from build123d import *

# Parameters (mm, degrees)
SKETCH1_W                 = 75
SKETCH1_H                 = 40
SKETCH1_R                 = 5
SKETCH1_R_2               = 1.7
SKETCH1_W_2               = 10
SKETCH1_H_2               = 20
BOSS_EXTRUDE1_DEPTH       = 3
CUT_EXTRUDE1_DEPTH        = 43.605750786
CUT_EXTRUDE1_DEPTH_BACK   = 43.605750786
SKETCH2_W                 = 67
SKETCH2_H                 = 28
BOSS_EXTRUDE3_DEPTH       = 110
BOSS_EXTRUDE3_DEPTH_BACK  = 3
SKETCH6_W                 = 67
SKETCH6_H                 = 11
CUT_EXTRUDE4_DEPTH        = 122.372360939
SKETCH7_W                 = 70
SKETCH7_H                 = 37
BOSS_EXTRUDE4_DEPTH       = 45
SKETCH8_W                 = 45
SKETCH8_H                 = 62
CUT_EXTRUDE6_DEPTH        = 29
SKETCH11_W                = 45
SKETCH11_H                = 4
CUT_EXTRUDE9_DEPTH        = 157.445677473
SKETCH9_W                 = 38
SKETCH9_H                 = 28.5
CUT_EXTRUDE10_DEPTH       = 204.024629048
SKETCH13_W                = 5
SKETCH13_H                = 38
BOSS_EXTRUDE5_DEPTH       = 32
SKETCH14_R                = 5
SKETCH14_R_2              = 1.7
CUT_EXTRUDE11_DEPTH       = 32
SKETCH15_W                = 165
SKETCH15_H                = 70
SKETCH15_W_2              = 157
SKETCH15_H_2              = 62
BOSS_EXTRUDE6_DEPTH       = 3
SKETCH16_W                = 20
SKETCH16_H                = 4.820648258
CUT_EXTRUDE12_DEPTH       = 159.626132778
SKETCH18_R                = 5
CUT_EXTRUDE14_DEPTH       = 159.626132778
MIRROR6_COPY_1_SKETCH_W   = 5
MIRROR6_COPY_1_SKETCH_H   = 38
MIRROR6_COPY_1_DEPTH      = 32
MIRROR6_COPY_2_SKETCH_R   = 5
MIRROR6_COPY_2_SKETCH_R_2 = 1.7
MIRROR6_COPY_2_DEPTH      = 32
SKETCH19_W                = 38
SKETCH19_H                = 3.5
CUT_EXTRUDE15_DEPTH       = 10
SKETCH20_R                = 1.2
CUT_EXTRUDE16_DEPTH       = 10
SKETCH21_W                = 10
SKETCH21_H                = 80
CUT_EXTRUDE17_DEPTH       = 184.330984833
SKETCH22_W                = 55
SKETCH22_H                = 80
CUT_EXTRUDE18_DEPTH       = 184.330984833
SKETCH23_W                = 67
SKETCH23_H                = 62
BOSS_EXTRUDE7_DEPTH       = 3
SKETCH24_R                = 10
SKETCH24_R_2              = 2.75
CUT_EXTRUDE19_DEPTH       = 111.707949127
SKETCH25_W                = 38
SKETCH25_H                = 64
CUT_EXTRUDE20_DEPTH       = 115
SKETCH26_W                = 49
SKETCH26_H                = 35
CUT_EXTRUDE21_DEPTH       = 32
SKETCH27_R                = 4.4
BOSS_EXTRUDE8_DEPTH       = 46


with BuildPart() as part:
    # Sketch1 → Boss-Extrude1 (new body)
    with BuildSketch(Plane(origin=(0, 0, 0), x_dir=(1, 0, 0), z_dir=(0, 1, 0))):
        Rectangle(SKETCH1_W, SKETCH1_H)
        with Locations(Location((-21, 0, 0), (0, 0, 270))):
            Circle(SKETCH1_R, mode=Mode.SUBTRACT)
        with Locations(Location((-30, 8.25, 0), (0, 0, 270))):
            Circle(SKETCH1_R_2, mode=Mode.SUBTRACT)
        with Locations(Location((-12, 8.25, 0), (0, 0, 270))):
            Circle(SKETCH1_R_2, mode=Mode.SUBTRACT)
        with Locations(Location((-12, -8.25, 0), (0, 0, 270))):
            Circle(SKETCH1_R_2, mode=Mode.SUBTRACT)
        with Locations(Location((-30, -8.25, 0), (0, 0, 270))):
            Circle(SKETCH1_R_2, mode=Mode.SUBTRACT)
        with Locations(Location((12, 8.25, 0), (0, 0, 90))):
            Circle(SKETCH1_R_2, mode=Mode.SUBTRACT)
        with Locations(Location((12, -8.25, 0), (0, 0, 90))):
            Circle(SKETCH1_R_2, mode=Mode.SUBTRACT)
        with Locations(Location((21, 0, 0), (0, 0, 90))):
            Circle(SKETCH1_R, mode=Mode.SUBTRACT)
        with Locations(Location((30, -8.25, 0), (0, 0, 90))):
            Circle(SKETCH1_R_2, mode=Mode.SUBTRACT)
        with Locations(Location((30, 8.25, 0), (0, 0, 90))):
            Circle(SKETCH1_R_2, mode=Mode.SUBTRACT)
        Rectangle(SKETCH1_W_2, SKETCH1_H_2, mode=Mode.SUBTRACT)
    extrude(amount=BOSS_EXTRUDE1_DEPTH)

    # Sketch2 → Cut-Extrude1 (cut, two sides: drawn at the far end of the back side and taken through both)
    with BuildSketch(Plane(origin=(0, 3, 0), x_dir=(1, 0, 0), z_dir=(0, 1, 0)).offset(-CUT_EXTRUDE1_DEPTH_BACK)):
        Rectangle(SKETCH2_W, SKETCH2_H)
    extrude(amount=CUT_EXTRUDE1_DEPTH + CUT_EXTRUDE1_DEPTH_BACK, mode=Mode.SUBTRACT)

    # Sketch3 → Boss-Extrude3 (add, two sides: drawn at the far end of the back side and taken through both)
    with BuildSketch(Plane(origin=(0, 3, 0), x_dir=(1, 0, 0), z_dir=(0, 1, 0)).offset(-BOSS_EXTRUDE3_DEPTH_BACK)):
        Polygon((37.5, -35), (37.5, -20), (33.5, -20), (-33.5, -20), (-37.5, -20), (-37.5, -35), align=None)
        Polygon((33.5, 20), (37.5, 20), (37.5, 35), (-37.5, 35), (-37.5, 20), (-33.5, 20), align=None)
        Polygon((37.5, -20), (37.5, 20), (33.5, 20), (33.5, 14), (33.5, -14), (33.5, -20), align=None)
        Polygon((-33.5, 14), (-33.5, 20), (-37.5, 20), (-37.5, -20), (-33.5, -20), (-33.5, -14), align=None)
    extrude(amount=BOSS_EXTRUDE3_DEPTH + BOSS_EXTRUDE3_DEPTH_BACK)

    # Sketch6 → Cut-Extrude4 (cut, through all)
    with BuildSketch(Plane(origin=(0, 3, 0), x_dir=(1, 0, 0), z_dir=(0, 1, 0))):
        with Locations((0, -25.5)):
            Rectangle(SKETCH6_W, SKETCH6_H)
        with Locations((0, 25.5)):
            Rectangle(SKETCH6_W, SKETCH6_H)
    extrude(amount=CUT_EXTRUDE4_DEPTH, mode=Mode.SUBTRACT)

    # Sketch7 → Boss-Extrude4 (add)
    with BuildSketch(Plane.ZY.offset(37.5)):
        with Locations((0, 94.5)):
            Rectangle(SKETCH7_W, SKETCH7_H)
    boss_extrude4 = extrude(amount=BOSS_EXTRUDE4_DEPTH)

    # Mirror2: Boss-Extrude4 across plane
    add(boss_extrude4.mirror(Plane(origin=(0, 0, 0), x_dir=(0, 0, 1), z_dir=(1, 0, 0))))

    # Sketch8 → Cut-Extrude6 (cut)
    with BuildSketch(Plane(origin=(0, 113, 0), x_dir=(1, 0, 0), z_dir=(0, 1, 0))):
        with Locations((-56, 0)):
            Rectangle(SKETCH8_W, SKETCH8_H)
        with Locations((56, 0)):
            Rectangle(SKETCH8_W, SKETCH8_H)
    extrude(amount=-CUT_EXTRUDE6_DEPTH, mode=Mode.SUBTRACT)

    # Sketch11 → Cut-Extrude9 (cut, through all)
    with BuildSketch(Plane.XY.offset(35)):
        with Locations((-60, 78)):
            Rectangle(SKETCH11_W, SKETCH11_H)
        with Locations((60, 78)):
            Rectangle(SKETCH11_W, SKETCH11_H)
    extrude(amount=-CUT_EXTRUDE9_DEPTH, mode=Mode.SUBTRACT)

    # Sketch9 → Cut-Extrude10 (cut, through all)
    with BuildSketch(Plane.ZY.offset(82.5)):
        with Locations((0, 98.25)):
            Rectangle(SKETCH9_W, SKETCH9_H)
    extrude(amount=-CUT_EXTRUDE10_DEPTH, mode=Mode.SUBTRACT)

    # Sketch13 → Boss-Extrude5 (add)
    with BuildSketch(Plane(origin=(0, 84, 0), x_dir=(1, 0, 0), z_dir=(0, 1, 0))):
        with Locations((-54.5, 0)):
            Rectangle(SKETCH13_W, SKETCH13_H)
    boss_extrude5 = extrude(amount=BOSS_EXTRUDE5_DEPTH)

    # Sketch14 → Cut-Extrude11 (cut)
    with BuildSketch(Plane.ZY.offset(57)):
        with Locations((0, 98.25)):
            Circle(SKETCH14_R)
        with Locations((-9, 106.5)):
            Circle(SKETCH14_R_2)
        with Locations((9, 106.5)):
            Circle(SKETCH14_R_2)
        with Locations((9, 90)):
            Circle(SKETCH14_R_2)
        with Locations((-9, 90)):
            Circle(SKETCH14_R_2)
    cut_extrude11 = extrude(amount=-CUT_EXTRUDE11_DEPTH, mode=Mode.SUBTRACT)

    # Mirror4: Boss-Extrude5, Cut-Extrude11 across plane
    add(boss_extrude5.mirror(Plane(origin=(0, 0, 0), x_dir=(0, 0, 1), z_dir=(1, 0, 0))))
    add(cut_extrude11.mirror(Plane(origin=(0, 0, 0), x_dir=(0, 0, 1), z_dir=(1, 0, 0))), mode=Mode.SUBTRACT)

    # Sketch15 → Boss-Extrude6 (add)
    with BuildSketch(Plane(origin=(0, 113, 0), x_dir=(1, 0, 0), z_dir=(0, 1, 0))):
        Rectangle(SKETCH15_W, SKETCH15_H)
        Rectangle(SKETCH15_W_2, SKETCH15_H_2, mode=Mode.SUBTRACT)
    extrude(amount=BOSS_EXTRUDE6_DEPTH)

    # Sketch16 → Cut-Extrude12 (cut, through all)
    with BuildSketch(Plane.XY.offset(35)):
        with Locations((0, 11.636111214)):
            Rectangle(SKETCH16_W, SKETCH16_H)
    extrude(amount=-CUT_EXTRUDE12_DEPTH, mode=Mode.SUBTRACT)

    # Sketch18 → Cut-Extrude14 (cut, through all)
    with BuildSketch(Plane.XY.offset(35)):
        with Locations((67.75, 100)):
            Circle(SKETCH18_R)
    cut_extrude14 = extrude(amount=-CUT_EXTRUDE14_DEPTH, mode=Mode.SUBTRACT)

    # Mirror5: Cut-Extrude14 across plane
    add(cut_extrude14.mirror(Plane(origin=(0, 0, 0), x_dir=(0, 0, 1), z_dir=(1, 0, 0))), mode=Mode.SUBTRACT)

    # Mirror6: Boss-Extrude5, Cut-Extrude11 across plane
    add(boss_extrude5.mirror(Plane.ZX.offset(116)))
    add(cut_extrude11.mirror(Plane.ZX.offset(116)), mode=Mode.SUBTRACT)

    # Mirror6 copy 1 sketch → Mirror6 copy 1 (add)
    with BuildSketch(Plane(origin=(0, 148, 0), x_dir=(-1, 0, 0), z_dir=(0, -1, 0))):
        with Locations((-54.5, 0)):
            Rectangle(MIRROR6_COPY_1_SKETCH_W, MIRROR6_COPY_1_SKETCH_H)
    extrude(amount=MIRROR6_COPY_1_DEPTH)

    # Mirror6 copy 2 sketch → Mirror6 copy 2 (cut)
    with BuildSketch(Plane(origin=(57, 232, 0), x_dir=(0, 0, 1), z_dir=(1, 0, 0))):
        with Locations((0, 98.25)):
            Circle(MIRROR6_COPY_2_SKETCH_R)
        with Locations((-9, 106.5)):
            Circle(MIRROR6_COPY_2_SKETCH_R_2)
        with Locations((9, 106.5)):
            Circle(MIRROR6_COPY_2_SKETCH_R_2)
        with Locations((9, 90)):
            Circle(MIRROR6_COPY_2_SKETCH_R_2)
        with Locations((-9, 90)):
            Circle(MIRROR6_COPY_2_SKETCH_R_2)
    extrude(amount=-MIRROR6_COPY_2_DEPTH, mode=Mode.SUBTRACT)

    # Sketch19 → Cut-Extrude15 (cut)
    with BuildSketch(Plane(origin=(82.5, 0, 0), x_dir=(0, 0, -1), z_dir=(1, 0, 0))):
        with Locations((0, 114.25)):
            Rectangle(SKETCH19_W, SKETCH19_H)
    cut_extrude15 = extrude(amount=-CUT_EXTRUDE15_DEPTH, mode=Mode.SUBTRACT)

    # Mirror7: Cut-Extrude15 across plane
    add(cut_extrude15.mirror(Plane(origin=(0, 0, 0), x_dir=(0, 0, 1), z_dir=(1, 0, 0))), mode=Mode.SUBTRACT)

    # Sketch20 → Cut-Extrude16 (cut)
    with BuildSketch(Plane(origin=(0, 3, 0), x_dir=(1, 0, 0), z_dir=(0, 1, 0))):
        with Locations(Location((-24, 17.5, 0), (0, 0, 270))):
            Circle(SKETCH20_R)
        with Locations(Location((-12, 17.5, 0), (0, 0, 270))):
            Circle(SKETCH20_R)
        with Locations(Location((12, 17.5, 0), (0, 0, 270))):
            Circle(SKETCH20_R)
        with Locations(Location((-24, -17.5, 0), (0, 0, 270))):
            Circle(SKETCH20_R)
        with Locations(Location((-12, -17.5, 0), (0, 0, 270))):
            Circle(SKETCH20_R)
        with Locations(Location((24, 17.5, 0), (0, 0, 270))):
            Circle(SKETCH20_R)
        with Locations(Location((12, -17.5, 0), (0, 0, 270))):
            Circle(SKETCH20_R)
        with Locations(Location((24, -17.5, 0), (0, 0, 270))):
            Circle(SKETCH20_R)
    extrude(amount=-CUT_EXTRUDE16_DEPTH, mode=Mode.SUBTRACT)

    # Sketch21 → Cut-Extrude17 (cut, through all)
    with BuildSketch(Plane.XY.offset(35)):
        with Locations((32.5, 40)):
            Rectangle(SKETCH21_W, SKETCH21_H)
        with Locations((-32.5, 40)):
            Rectangle(SKETCH21_W, SKETCH21_H)
    extrude(amount=-CUT_EXTRUDE17_DEPTH, mode=Mode.SUBTRACT)

    # Sketch22 → Cut-Extrude18 (cut, through all)
    with BuildSketch(Plane.XY.offset(35)):
        with Locations((0, 40)):
            Rectangle(SKETCH22_W, SKETCH22_H)
    extrude(amount=-CUT_EXTRUDE18_DEPTH, mode=Mode.SUBTRACT)

    # Sketch23 → Boss-Extrude7 (add)
    with BuildSketch(Plane.XZ.offset(-80)):
        Rectangle(SKETCH23_W, SKETCH23_H)
    extrude(amount=-BOSS_EXTRUDE7_DEPTH)

    # Sketch24 → Cut-Extrude19 (cut, through all)
    with BuildSketch(Plane(origin=(0, 83, 0), x_dir=(1, 0, 0), z_dir=(0, 1, 0))):
        with Locations(Location((0, 0, 0), (0, 0, 270))):
            Circle(SKETCH24_R)
        with Locations(Location((-20, 19, 0), (0, 0, 270))):
            Circle(SKETCH24_R_2)
        with Locations(Location((-20, -19, 0), (0, 0, 270))):
            Circle(SKETCH24_R_2)
        with Locations(Location((20, -19, 0), (0, 0, 90))):
            Circle(SKETCH24_R_2)
        with Locations(Location((20, 19, 0), (0, 0, 90))):
            Circle(SKETCH24_R_2)
    extrude(amount=-CUT_EXTRUDE19_DEPTH, mode=Mode.SUBTRACT)

    # Sketch25 → Cut-Extrude20 (cut)
    with BuildSketch(Plane(origin=(57, 0, 0), x_dir=(0, 0, -1), z_dir=(1, 0, 0))):
        with Locations((0, 116)):
            Rectangle(SKETCH25_W, SKETCH25_H)
    extrude(amount=-CUT_EXTRUDE20_DEPTH, mode=Mode.SUBTRACT)

    # Sketch26 → Cut-Extrude21 (cut)
    with BuildSketch(Plane(origin=(0, 116, 0), x_dir=(1, 0, 0), z_dir=(0, 1, 0))):
        with Locations((58, -17.5)):
            Rectangle(SKETCH26_W, SKETCH26_H)
    cut_extrude21 = extrude(amount=-CUT_EXTRUDE21_DEPTH, mode=Mode.SUBTRACT)

    # Mirror8: Cut-Extrude21 across plane
    add(cut_extrude21.mirror(Plane(origin=(0, 0, 0), x_dir=(0, 0, 1), z_dir=(1, 0, 0))), mode=Mode.SUBTRACT)

    # Sketch27 → Boss-Extrude8 (add)
    with BuildSketch(Plane(origin=(0, 84, 0), x_dir=(1, 0, 0), z_dir=(0, 1, 0))):
        with Locations(Location((65.5, -15, 0), (0, 0, 90))):
            Circle(SKETCH27_R)
    boss_extrude8 = extrude(amount=BOSS_EXTRUDE8_DEPTH)

    # Mirror9: Boss-Extrude8 across plane
    add(boss_extrude8.mirror(Plane(origin=(0, 0, 0), x_dir=(0, 0, 1), z_dir=(1, 0, 0))))


solid = part.part
Verification items for the finished model (mm, model axes). A direction names the side the tool comes from. Give positions to 0.01 mm unless a question says otherwise; leave off trailing zeros. Order: outer loops, then holes, each group sorted by start corner. A loop starts at its lowest first (then second) coordinate and runs counter-clockwise, first axis right, second up. Notation, with made-up numbers: (66.25, 30) -> (70.25, 30) arc R23 ccw to (70.25, 61) -> close; hole circle Ø7 at (-4, 54.25). An arc over 180 degrees is marked (long way). Answer as CSV lines item,"result".
Q1. Sectioned sample at D-D on x = 67.75. Record the cut outline in (y, z).
Solutions:
outline,"(80, -35) -> (95, -35) -> (95, -31) -> (84, -31) -> (84, 11.22) -> (130, 11.22) -> (130, 18.78) -> (84, 18.78) -> (84, 35) -> (80, 35) -> close; (105, -35) -> (116, -35) -> (116, -31) -> (105, -31) -> close"
Q2. Sectioned sample at B-B on y = 86.5. Record the cut outline in (x, z).
Solutions:
outline,"(-82.5, -35) -> (82.5, -35) -> (82.5, -19) -> (78.5, -19) -> (78.5, -31) -> (-78.5, -31) -> (-78.5, -19) -> (-82.5, -19) -> close; circle Ø8.8 at (-65.5, 15); (-33.5, 31) -> (33.5, 31) -> (33.5, 35) -> (-33.5, 35) -> close; circle Ø8.8 at (65.5, 15)"
Q3. Sectioned sample at A-A on x = -20. Record the cut outline in (y, z).
Solutions:
outline,"(80, -35) -> (116, -35) -> (116, -31) -> (83, -31) -> (83, -21.75) -> (80, -21.75) -> close; (80, -16.25) -> (83, -16.25) -> (83, 16.25) -> (80, 16.25) -> close; (80, 21.75) -> (83, 21.75) -> (83, 31) -> (116, 31) -> (116, 35) -> (80, 35) -> close"
Q4. Release check for a two-part mould opening along Z. For faces 5 (the flat face through (-1, 94, 35)), 6 (the flat face through (-82.5, 93, -21)), 7 (the cylindrical face through (-17.273, 81.521, 18.642)), 8 (the flat face through (-8, 83, 7)) record: +Z half, -Z half, draft (parallel to the pull), parting line (faces both ways), or undercut.
Solutions:
face 5,"+Z half"
face 6,"draft"
face 7,"undercut"
face 8,"undercut"
Q5. Depth check by flat-ended pin: pin 1 (24.5 mm diameter, centred on x = 48.5, z = 8.5, fed in from +Y); pin 2 (8 mm diameter, centred on x = -19.5, z = -28.5, fed in from +Y); pin 3 (7 mm diameter, centred on x = -20, z = -19, fed in from +Y). Enter the tip coordinate at first touch or a pass-through.
Solutions:
pin 1,"stops at y = 84"
pin 2,"stops at y = 116"
pin 3,"stops at y = 83"
Q6. Access from +Z, -Z, +X, -X, +Y, -Y to the whole of each face (thin tool, end or side, straight path). Record for faces 1 (the flat face through (-81, 100, -19)), 2 (the cylindrical face through (-66.67, 95.12, -32.97)), 3 (the flat face through (82.5, 93, -21)), 4 (the flat face through (-78.5, 100, -25)).
Solutions:
face 1,"+Z, +X, -X, +Y"
face 2,"-Z"
face 3,"+Z, -Z, +X, +Y, -Y"
face 4,"+Z, +Y"
Q7. Sectioned sample at C-C on y = 100. Record the cut outline in (x, z), plus the area to 3 significant figures.
Solutions:
outline,"(-82.5, -35) -> (-72.75, -35) -> (-72.75, -31) -> (-78.5, -31) -> (-78.5, -19) -> (-82.5, -19) -> close; circle Ø8.8 at (-65.5, 15); (-62.75, -35) -> (62.75, -35) -> (62.75, -31) -> (-62.75, -31) -> close; (-33.5, 31) -> (33.5, 31) -> (33.5, 35) -> (-33.5, 35) -> close; circle Ø8.8 at (65.5, 15); (72.75, -35) -> (82.5, -35) -> (82.5, -19) -> (78.5, -19) -> (78.5, -31) -> (72.75, -31) -> close"
area,"1,070 mm²"
Q8. Scan lines: probe 1 along X at (y, z) = (82.25, -19); probe 2 along Z at (x, y) = (20, 82); probe 3 along Y at (x, z) = (-67.75, -33.3). Record each from-to range of solid material in increasing order.
Solutions:
probe 1,"x = -82.5 to -22.75, -17.25 to 17.25, 22.75 to 82.5"
probe 2,"z = -35 to -21.75, -16.25 to 16.25, 21.75 to 35"
probe 3,"y = 80 to 95, 105 to 116"
